Check sheet for the drawn part. Datum: minimum x, y, z corner. Units: mm. Coordinates: 2 decimals unless noted, no trailing zeros. Order: outer loops, then holes, each group sorted by start corner. A loop starts at its lowest first (then second) coordinate and runs counter-clockwise, first axis right, second up. Notation, with made-up numbers: (-35.5, 85.25) - (5.5, 85.25) arc R28 cw to (5.5, 117.25) - close; hole circle Ø5 at (-18, -6). An arc over 180 degrees is marked (long way). One line per item, written item: value. Start each with the question number.
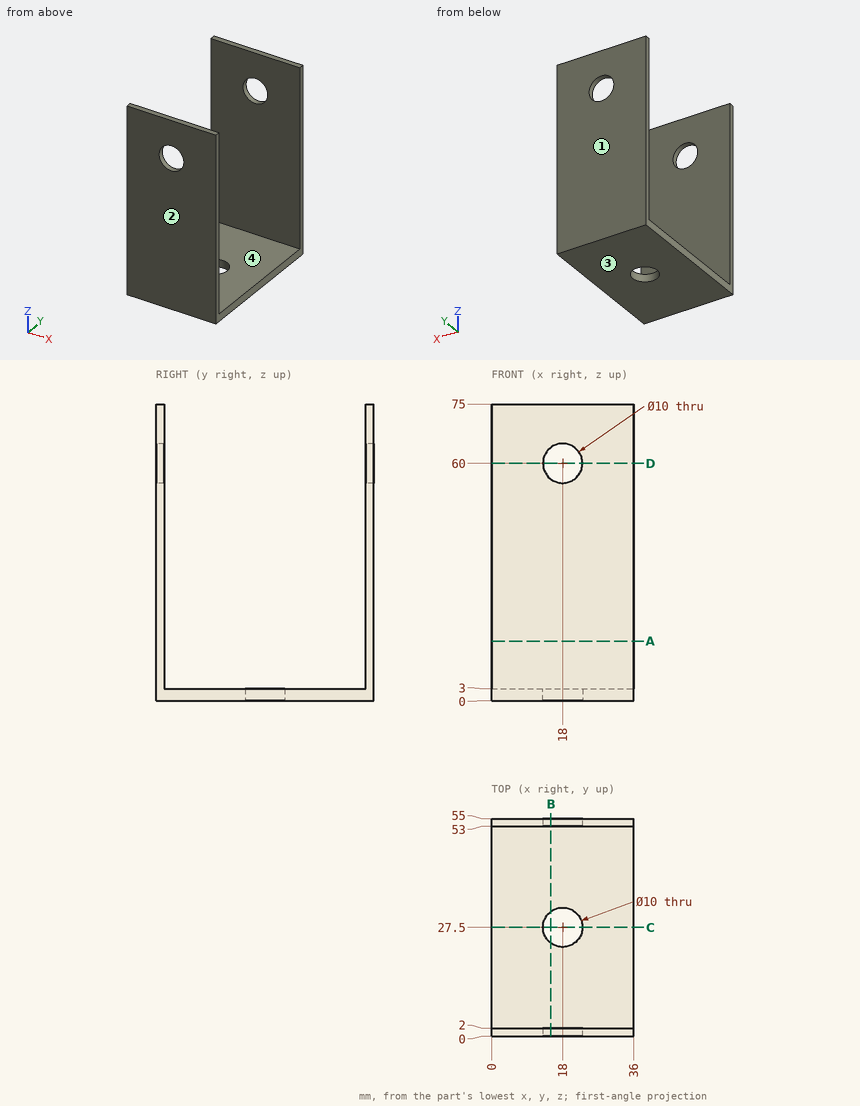
Q1. Cross-section at A-A, the plane z = 15. Enter the section's corners in (x, y), and give its area (3 significant figures).
Q2. Cross-section at B-B, the plane x = 15. Enter the section's corners in (y, z), and give its area (3 significant figures).
Q3. Material ranges on probe 1 along Y at (x, z) = (18, 1.7); probe 2 along Y at (x, z) = (6.5, 51); probe 3 along Z at (x, y) = (18, 53.8), recorded low to high.
Q4. Cross-section at D-D, the plane z = 60. Enter the section's corners in (x, y), and give its area (3 significant figures).
Q5. Gauge pin test, flat end, axial feed: P1, Ø2, axis at x = 22, y = 26, coming from the +Z side. Record the tip position at first contact, or that the pin passes through.
Q6. Release check for a two-part mould opening along Y. For the marked faces 1, 2, 3 and 4 record: released by +Y, released by -Y, zero draft, split by the parting line, or undercut.
Q7. Cross-section at C-C, the plane y = 27.5. Enter the section's corners in (x, z).
Check result:
1. outline: (0, 0) - (36, 0) - (36, 2) - (0, 2) - close; (0, 53) - (36, 53) - (36, 55) - (0, 55) - close
1. area: 144 mm2
2. outline: (0, 0) - (23.5, 0) - (23.5, 3) - (2, 3) - (2, 56) - (0, 56) - close; (0, 64) - (2, 64) - (2, 75) - (0, 75) - close; (31.5, 0) - (55, 0) - (55, 56) - (53, 56) - (53, 3) - (31.5, 3) - close; (53, 64) - (55, 64) - (55, 75) - (53, 75) - close
2. area: 397 mm2
3. probe 1: y = 0 to 22.5, 32.5 to 55
3. probe 2: y = 0 to 2, 53 to 55
3. probe 3: z = 0 to 55, 65 to 75
4. outline: (0, 0) - (13, 0) - (13, 2) - (0, 2) - close; (0, 53) - (13, 53) - (13, 55) - (0, 55) - close; (23, 0) - (36, 0) - (36, 2) - (23, 2) - close; (23, 53) - (36, 53) - (36, 55) - (23, 55) - close
4. area: 104 mm2
5. P1: stops at z = 3
6. face 1: released by +Y
6. face 2: released by -Y
6. face 3: zero draft
6. face 4: undercut
7. outline: (0, 0) - (13, 0) - (13, 3) - (0, 3) - close; (23, 0) - (36, 0) - (36, 3) - (23, 3) - close
